Here's how the part is built. I have some questions about the finished solid (model axes, mm). Coordinates: 2 decimals unless noted, no trailing zeros. Write each loop counter-clockwise with the first axis right and the second up, starting at its lowest first coordinate (ties: lowest second). Pieces come first, ordered by that corner, then holes.
(1) For pin 1 Ø6.5 at (x, z) = (-10, 55) entering from -Y, with a flat end and sliding along its axis, tell me the tip position at first contact or that it passes through.
(2) Imagine slicing it at C-C, the plane x = -10.75. List the corners of the cut face in (y, z) for me.
(3) Please list where these lines run through material, in increasing order: probe 1 along Z at (x, y) = (-10, 3.1); probe 2 along Z at (x, y) = (-10.5, 1.4); probe 3 along X at (y, z) = (3.3, 68).
(4) Imagine slicing it at A-A, the plane z = 55. List the corners of the cut face in (x, y) for me.
(5) Imagine slicing it at B-B, the plane y = 2.5. List the corners of the cut face in (x, z) for me, plus the area to 3 significant figures.
Autodesk Inventor part; units mm, degrees
ref_plane "YZ Plane" through (0, 0, 0) normal (1, 0, 0) x (0, 1, 0)
ref_plane "XZ Plane" through (0, 0, 0) normal (0, 1, 0) x (-1, 0, 0)
ref_plane "XY Plane" through (0, 0, 0) normal (0, 0, 1) x (1, 0, 0)
sketch "Sketch4" plane through (0, 0, 0) normal (0, 1, 0) x (-1, 0, 0)
  line L0 (0, 0) -> (20, 0)
  line L1 (20, 0) -> (20, 80)
  line L2 (20, 80) -> (0, 80)
  line L3 (0, 80) -> (0, 0)
  circle A0 centre (-8.1929, 3.0927) radius 2.5
  dimension "d0" = 80
  dimension "d3" = 20
extrude "Extrusion1" add sketch "Sketch4" along normal blind 5 contours L3 L2 L1 L0
sketch "Sketch5" plane through (0, 0, 0) normal (0, -1, 0) x (1, 0, 0)
  line L0 (0, 0) -> (-20, 0)
  line L1 (0, 80) -> (0, 0)
  line L2 (-20, 80) -> (0, 80)
  line L3 (-20, 0) -> (-20, 80)
  circle A0 centre (-10, 10) radius 2.5
  circle A1 centre (-10, 70) radius 2.5
  circle A2 centre (-10, 55) radius 2.5
  dimension "d5" = 5
  dimension "d6" = 5
  dimension "d7" = 10
  dimension "d8" = 10
  dimension "d9" = 10
  dimension "d10" = 10
  dimension "d13" = 5
  dimension "d17" = 15
extrude "Extrusion3" cut sketch "Sketch5" against normal through all contours A0 | A1 | A2
properties part number "holdersupport" material "Wood (Birch)"
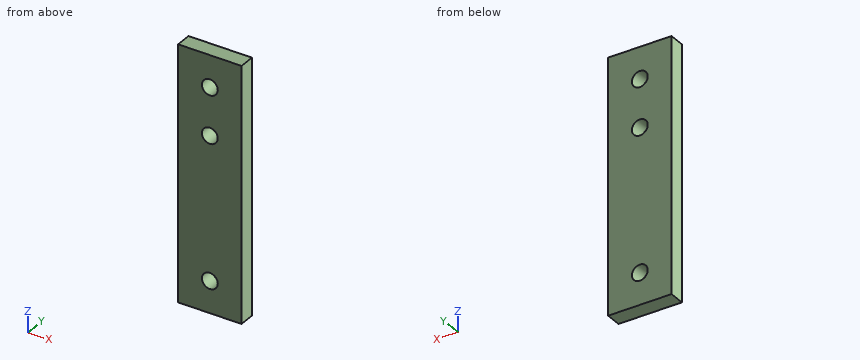
Recorded:
1. pin 1: stops at y = 0
2. outline: (0, 0) - (5, 0) - (5, 7.62) - (0, 7.62) - close; (0, 12.38) - (5, 12.38) - (5, 52.62) - (0, 52.62) - close; (0, 57.38) - (5, 57.38) - (5, 67.62) - (0, 67.62) - close; (0, 72.38) - (5, 72.38) - (5, 80) - (0, 80) - close
3. probe 1: z = 0 to 7.5, 12.5 to 52.5, 57.5 to 67.5, 72.5 to 80
3. probe 2: z = 0 to 7.55, 12.45 to 52.55, 57.45 to 67.55, 72.45 to 80
3. probe 3: x = -20 to -11.5, -8.5 to 0
4. outline: (-20, 0) - (-12.5, 0) - (-12.5, 5) - (-20, 5) - close; (-7.5, 0) - (0, 0) - (0, 5) - (-7.5, 5) - close
5. outline: (-20, 0) - (0, 0) - (0, 80) - (-20, 80) - close; hole circle Ø5 at (-10, 10); hole circle Ø5 at (-10, 55); hole circle Ø5 at (-10, 70)
5. area: 1,540 mm2
